```python
from build123d import *

# Parameters (mm, degrees)
F1_DEPTH  = 25.4
F2_DEPTH  = 50.8
F9_R      = 6.604
F10_DEPTH = 111.76
F11_R     = 38.1
F12_DEPTH = 10.668
F13_R     = 5.08


with BuildPart() as f1:
    # F0 (on Top) → F1 (new body)
    with BuildSketch(Plane.XY):
        with BuildLine():
            Line((0, -114.0008171796), (0, 114.599125499))
            ThreePointArc((0, 114.599125499), (-114.2190565937, 0.2991541597), (0, -114.0008171796))
        make_face()
    extrude(amount=F1_DEPTH)

    # F0 (on Top) → F2 (join)
    with BuildSketch(Plane.XY):
        with BuildLine():
            ThreePointArc((0, -114.0008171796), (-114.2190565937, 0.2991541597), (0, 114.599125499))
            Line((0, 114.599125499), (-0.0044968559, 120.9491239067))
            ThreePointArc((-0.0044968559, 120.9491239067), (-120.5690565937, 0.2991541597), (-0.0044968559, -120.3508155874))
            Line((-0.0044968559, -120.3508155874), (0, -114.0008171796))
        make_face()
    extrude(amount=F2_DEPTH)

    # F1_face (on face) → F5 section 0
    with BuildSketch(Plane(origin=(-48.4732263634, 0.2991541597, 25.4), x_dir=(1, 0, 0), z_dir=(0, 0, 1))):
        with BuildLine():
            Line((48.4732263634, -114.2999713393), (48.4732263634, 114.2999713393))
            ThreePointArc((48.4732263634, 114.2999713393), (-65.7458302303, 0), (48.4732263634, -114.2999713393))
        make_face()
    # F4 (on offset) → F5 section 1
    with BuildSketch(Plane.XY.offset(111.76)):
        with BuildLine():
            Line((0, 0), (0, 25.4))
            ThreePointArc((0, 25.4), (-25.4, 0), (0, -25.4))
            Line((0, -25.4), (0, 0))
        make_face()
    loft()

    # F9 (on Top) → F10 (cut)
    with BuildSketch(Plane.XY):
        Circle(F9_R)
    extrude(amount=F10_DEPTH, mode=Mode.SUBTRACT)

    # F11 (on offset) → F12 (cut)
    with BuildSketch(Plane.XY.offset(50.8)):
        Circle(F11_R)
    extrude(amount=F12_DEPTH, mode=Mode.SUBTRACT)

    # F13
    f13_edges = [f1.edges().sort_by_distance(p)[0] for p in [
        (-38.1, 0, 61.468),
        (-38.1, 0, 50.8),
    ]]
    fillet(f13_edges, radius=F13_R)


solid = f1.part
```
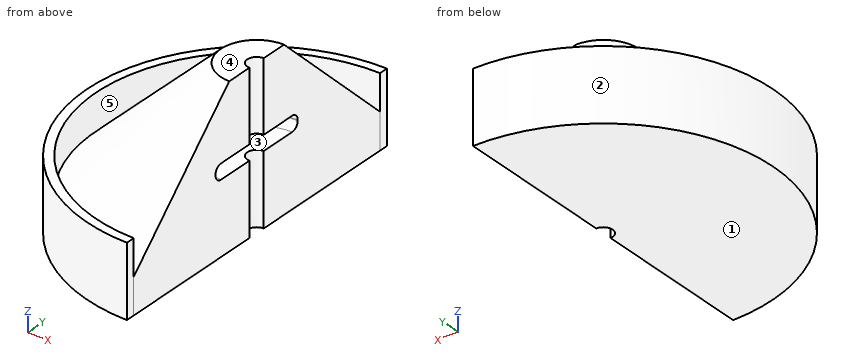
Design review of the part built by this model. Coordinates are the model's own, in mm. Face numbers are marked on the shaded views. A direction names the side the tool comes from. Coordinates: 2 decimals unless noted, no trailing zeros. Write each loop counter-clockwise with the first axis right and the second up, starting at its lowest first coordinate (ties: lowest second). Pieces come first, ordered by that corner, then holes.
1) To check wall thickness, follow L1, parallel to Y at x = -53, z = 39.5; L2, parallel to Y at x = -38.5, z = 28; L3, parallel to Z at x = -113, y = -32. State the ranges of each line that lie inside material, in increasing order.
2) Machinability: for the marked faces 4 and 5, which of the approach directions +Z, -Z, +X, -X, +Y, -Y give a long, thin tool a straight path to every point of the face, cutting with its end or side? Answer none if there is none.
3) Insertion check: pin 1 (10 mm diameter, centred on x = -23, y = -9.5, fed in from -Z); pin 2 (1 mm diameter, centred on x = -56, y = -56.5, fed in from +Z). Each pin has a flat end and moves straight along its axis. Give the tip position at first contact, or say it passes through.
4) Mouldability with a two-part tool opening along Y and no side actions: class the marked faces 1, 2 and 3 as +Y half, -Y half, draft (parallel to the pull), parting line (faces both ways), or undercut.
5) Add section A-A (z = 16). Write out the cut boundary in (x, y), plus the area to 3 significant figures.
Check result:
1. L1: y = -108.05 to -100.93, -84.25 to 84.75, 101.53 to 108.65
1. L2: y = -114.02 to -107.29, -104.45 to 105.04, 107.89 to 114.61
1. L3: z = 0 to 50.8
2. face 4: +Z, +X, -X, +Y, -Y
2. face 5: +Z
3. pin 1: stops at z = 0
3. pin 2: stops at z = 59.48
4. face 1: draft
4. face 2: parting line
4. face 3: undercut
5. outline: (0, -120.35) - (0, -114) - (0, -6.6) arc R6.6 cw to (0, 6.6) - (0, 114.6) - (0, 120.95) arc R120.65 ccw to start
5. area: 22,800 mm2
